from build123d import *

# Parameters (mm, degrees)
F0_R     = 5.75
F0_R_2   = 5
F1_DEPTH = 1
F0_R_3   = 3.5
F0_R_4   = 2.5
F0_R_5   = 1.5
F2_DEPTH = 4
F3_R     = 0.3
F4_R     = 2.65
F4_R_2   = 2.5
F5_DEPTH = 0.2
F4_R_3   = 4
F4_R_4   = 3.5
F6_DEPTH = 0.3
F7_DEPTH = 0.2


with BuildPart() as f1:
    # F0 (on Front) → F1 (new body)
    with BuildSketch(Plane.XZ):
        Circle(F0_R)
        Circle(F0_R_2, mode=Mode.SUBTRACT)
    extrude(amount=F1_DEPTH)

    # F0 (on Front) → F2 (join)
    with BuildSketch(Plane.XZ):
        Circle(F0_R_2)
        Circle(F0_R_3, mode=Mode.SUBTRACT)
        Circle(F0_R_3)
        Circle(F0_R_4, mode=Mode.SUBTRACT)
        Circle(F0_R_4)
        Circle(F0_R_5, mode=Mode.SUBTRACT)
    extrude(amount=F2_DEPTH)

    # F3
    f3_edges = [f1.edges().sort_by_distance(p)[0] for p in [
        (-5, -4, 0),
        (-1.5, -4, 0),
        (-1.5, 0, 0),
    ]]
    fillet(f3_edges, radius=F3_R)

    # F4 (on face) → F5 (cut)
    with BuildSketch(Plane.XZ.offset(4)):
        Circle(F4_R)
        Circle(F4_R_2, mode=Mode.SUBTRACT)
    extrude(amount=-F5_DEPTH, mode=Mode.SUBTRACT)

    # F4 (on face) → F6 (cut)
    with BuildSketch(Plane.XZ.offset(4)):
        Circle(F4_R_3)
        Circle(F4_R_4, mode=Mode.SUBTRACT)
    extrude(amount=-F6_DEPTH, mode=Mode.SUBTRACT)

    # F0 (on Front) → F7 (cut)
    with BuildSketch(Plane.XZ):
        Circle(F0_R_3)
        Circle(F0_R_4, mode=Mode.SUBTRACT)
    extrude(amount=F7_DEPTH, mode=Mode.SUBTRACT)


solid = f1.part
Geometry: final body of the model. Coordinates: model frame, mm. A direction names the side the tool comes from. Coordinates: 2 decimals unless noted, no trailing zeros. Order: outer loops, then holes, each group sorted by start corner. A loop starts at its lowest first (then second) coordinate and runs counter-clockwise, first axis right, second up.
1) Ray query, probe 1 along Z at (x, y) = (3, -3.3); probe 2 along Y at (x, z) = (4.75, 0); probe 3 along Z at (x, y) = (0, -0.1). Return the intervals inside material, ascending.
Result sheet:
probe 1: z = -4 to 4
probe 2: y = -4 to 0
probe 3: z = -5.75 to -3.5, -2.5 to -1.58, 1.58 to 2.5, 3.5 to 5.75
2) Section B-B (y = -2.4). Return loops of the section in (x, z).
Result sheet:
outline: circle Ø10 at (0, 0); hole circle Ø3 at (0, 0)
3) Set-up query: faces 1 (the flat face through (2, -4, 4)), 2 (the flat face through (2, -0.2, -2)), 3 (the flat face through (-2, -1, 5)). Return all of +Z, -Z, +X, -X, +Y, -Y with unobstructed straight access to the full face (end or side cutting, diameter ignored); none if empty.
Result sheet:
face 1: +Z, -Z, +X, -X, -Y
face 2: +Y
face 3: -Y
4) Draft query along Z for faces 4 (the flat face through (0, 0, -4)), 5 (the cylindrical face through (-1.5, -1.98, 0.07)), 6 (the cylindrical face through (-1.08, -2.33, -4.88)). Return one class per face: released by +Z, released by -Z, zero draft, split by the parting line, or undercut.
Result sheet:
face 4: zero draft
face 5: undercut
face 6: split by the parting line
5) Section A-A (y = -0.7). Return loops of the section in (x, z).
Result sheet:
outline: circle Ø11.5 at (0, 0); hole circle Ø3 at (0, 0)
6) First-contact query: P1, Ø1, axis at x = -3.5, y = -2.5, coming from the +Z side; P2, Ø2, axis at y = -1.5, z = -4, coming from the +X side; P3, Ø1.8, axis at x = 0, z = 0, coming from the -Y side. Flat tips, straight axial feed; report the tip coordinate or a pass-through.
Result sheet:
P1: stops at z = 4
P2: stops at x = 4.82
P3: passes through
